CAD build for the part. Positions are in the model's coordinates, mm. Round coordinates to 2 decimals unless told otherwise and drop trailing zeros. Loops run counter-clockwise (first coordinate to the right, second up) from the corner with the lowest first, then second, coordinate; pieces in that order, holes last. Notation, with made-up numbers: M -15.5,28 L 36.5,28 A21 cw 36.5,33 Z; hole C 54,77 d11. An arc over 180 degrees is marked long. Use a Markdown table: item, result. Add a question column.
(1) Flat gauge pins, fed straight in: P1, Ø3, axis at x = 11, y = 10, coming from the +Z side; P2, Ø0.9, axis at y = 56.5, z = 1.5, coming from the -X side. Where does each tip first touch, or does it go through?
(2) Band-saw the part on A-A, the plane x = 3. Write the cut outline in (y, z), and give its area (3 significant figures).
(3) Wall check: L1, parallel to Y at x = 32, z = 0.9; L2, parallel to Y at x = 11, z = 2.4; L3, parallel to Y at x = 31, z = 2.6. Give the ranges that are in metal, low to high.
(4) Band-saw the part on B-B, the plane z = 2.15. Write the cut outline in (x, y).
from build123d import *

# Parameters (mm, degrees)
SKETCH1_W                    = 42
SKETCH1_H                    = 260
BOSS_EXTRUDE1_DEPTH          = 3
M3_CLEARANCE_HOLE1_OUTLINE_R = 1.6
M3_CLEARANCE_HOLE1_DEPTH     = 3
SKETCH4_W                    = 20
SKETCH4_H                    = 30
CUT_EXTRUDE1_DEPTH           = 10


# Read off the part's stored shape, not the designer's step: M3 Clearance Hole1
with BuildPart() as part:
    # Sketch1 → Boss-Extrude1 (new body)
    with BuildSketch(Plane.XY):
        with Locations((21, 130)):
            Rectangle(SKETCH1_W, SKETCH1_H)
    extrude(amount=BOSS_EXTRUDE1_DEPTH)

    # M3 Clearance Hole1 outline → M3 Clearance Hole1 (cut)
    with BuildSketch(Plane.XY):
        with Locations((32, 130)):
            Circle(M3_CLEARANCE_HOLE1_OUTLINE_R)
        with Locations((32, 10)):
            Circle(M3_CLEARANCE_HOLE1_OUTLINE_R)
        with Locations((32, 250)):
            Circle(M3_CLEARANCE_HOLE1_OUTLINE_R)
        with Locations((11, 10)):
            Circle(M3_CLEARANCE_HOLE1_OUTLINE_R)
    extrude(amount=M3_CLEARANCE_HOLE1_DEPTH, mode=Mode.SUBTRACT)

    # Sketch4 → Cut-Extrude1 (cut)
    with BuildSketch(Plane.XY.offset(3)):
        with Locations((10, 55)):
            Rectangle(SKETCH4_W, SKETCH4_H)
    extrude(amount=-CUT_EXTRUDE1_DEPTH, mode=Mode.SUBTRACT)


solid = part.part
Return value:
| question | item | result |
|---|---|---|
| 1 | P1 | through |
| 1 | P2 | x = 20 |
| 2 | outline | M 0,0 L 40,0 L 40,3 L 0,3 Z; M 70,0 L 260,0 L 260,3 L 70,3 Z |
| 2 | area | 690 mm^2 |
| 3 | L1 | 0 to 8.4, 11.6 to 128.4, 131.6 to 248.4, 251.6 to 260 |
| 3 | L2 | 0 to 8.4, 11.6 to 40, 70 to 260 |
| 3 | L3 | 0 to 8.75, 11.25 to 128.75, 131.25 to 248.75, 251.25 to 260 |
| 4 | outline | M 0,0 L 42,0 L 42,260 L 0,260 L 0,70 L 20,70 L 20,40 L 0,40 Z; hole C 11,10 d3.2; hole C 32,10 d3.2; hole C 32,130 d3.2; hole C 32,250 d3.2 |
